```python
from build123d import *

# Parameters (mm, degrees)
SKETCH1_R           = 40
SKETCH1_W           = 12.2
SKETCH1_H           = 22.7
BOSS_EXTRUDE1_DEPTH = 16.35
SKETCH3_W           = 5
SKETCH3_H           = 34.105
CUT_EXTRUDE1_DEPTH  = 7
SKETCH4_R           = 1.75
CUT_EXTRUDE2_DEPTH  = 8
SKETCH2_R           = 40
SKETCH2_W           = 12.2
SKETCH2_H           = 32.25
BOSS_EXTRUDE2_DEPTH = 8.3
SKETCH5_R           = 1
CUT_EXTRUDE3_DEPTH  = 8
SKETCH6_R           = 40
BOSS_EXTRUDE3_DEPTH = 2.5
BOSS_EXTRUDE4_DEPTH = 31.05
CUT_EXTRUDE4_START  = -8
SKETCH8_R           = 1.75
CUT_EXTRUDE4_DEPTH  = 8
FILLET1_R           = 1


with BuildPart() as part:
    # Sketch1 → Boss-Extrude1 (new body)
    with BuildSketch(Plane(origin=(0, 0, 0), x_dir=(1, 0, 0), z_dir=(0, 1, 0))):
        with Locations(Location((0, 0, 0), (0, 0, 270))):
            Circle(SKETCH1_R)
        with Locations((0, 5.455)):
            Rectangle(SKETCH1_W, SKETCH1_H, mode=Mode.SUBTRACT)
    extrude(amount=BOSS_EXTRUDE1_DEPTH)

    # Sketch3 → Cut-Extrude1 (cut)
    with BuildSketch(Plane.XZ):
        with Locations((0, 22.9475)):
            Rectangle(SKETCH3_W, SKETCH3_H)
    extrude(amount=-CUT_EXTRUDE1_DEPTH, mode=Mode.SUBTRACT)

    # Sketch4 → Cut-Extrude2 (cut)
    with BuildSketch(Plane.XZ):
        with Locations(Location((-15.556349186, 15.556349186, 0), (0, 0, 270))):
            Circle(SKETCH4_R)
        with Locations(Location((15.556349186, 15.556349186, 0), (0, 0, 270))):
            Circle(SKETCH4_R)
        with Locations(Location((15.556349186, -15.556349186, 0), (0, 0, 270))):
            Circle(SKETCH4_R)
        with Locations(Location((-15.556349186, -15.556349186, 0), (0, 0, 270))):
            Circle(SKETCH4_R)
    extrude(amount=-CUT_EXTRUDE2_DEPTH, mode=Mode.SUBTRACT)

    # Sketch2 → Boss-Extrude2 (add)
    with BuildSketch(Plane(origin=(0, 16.35, 0), x_dir=(1, 0, 0), z_dir=(0, 1, 0))):
        with Locations(Location((0, 0, 0), (0, 0, 266.416678302))):
            Circle(SKETCH2_R)
        with Locations((0, 5.455)):
            Rectangle(SKETCH2_W, SKETCH2_H, mode=Mode.SUBTRACT)
    extrude(amount=BOSS_EXTRUDE2_DEPTH)

    # Sketch5 → Cut-Extrude3 (cut)
    with BuildSketch(Plane(origin=(0, 16.35, 0), x_dir=(1, 0, 0), z_dir=(0, 1, 0))):
        with Locations(Location((0, 19.58, 0), (0, 0, 270))):
            Circle(SKETCH5_R)
        with Locations(Location((0, -8.67, 0), (0, 0, 90))):
            Circle(SKETCH5_R)
    extrude(amount=-CUT_EXTRUDE3_DEPTH, mode=Mode.SUBTRACT)

    # Sketch6 → Boss-Extrude3 (add)
    with BuildSketch(Plane(origin=(0, 24.65, 0), x_dir=(1, 0, 0), z_dir=(0, 1, 0))):
        with Locations(Location((0, 0, 0), (0, 0, 266.416678302))):
            Circle(SKETCH6_R)
        with BuildLine():
            Line((6.1, 12.043255374), (6.1, 21.58))
            Line((6.1, 21.58), (-6.1, 21.58))
            Line((-6.1, 21.58), (-6.1, 12.043255374))
            ThreePointArc((-6.1, 12.043255374), (0, -13.5), (6.1, 12.043255374))
        make_face(mode=Mode.SUBTRACT)
    extrude(amount=BOSS_EXTRUDE3_DEPTH)

    # Sketch7 → Boss-Extrude4 (add)
    with BuildSketch(Plane(origin=(0, 27.15, 0), x_dir=(1, 0, 0), z_dir=(0, 1, 0))):
        with BuildLine():
            ThreePointArc((-4.790054945, -12.621623256), (-13.48100084, -0.715972321), (-6.1, 12.043255374))
            Line((-6.1, 12.043255374), (-6.1, 21.58))
            Line((-6.1, 21.58), (6.1, 21.58))
            Line((6.1, 21.58), (6.1, 12.043255374))
            ThreePointArc((6.1, 12.043255374), (13.480999281, -0.716001663), (4.79, -12.621644108))
            Line((4.79, -12.621644108), (4.79, -13))
            Line((4.79, -13), (10.89, -13))
            Line((10.89, -13), (10.89, -14.6))
            Line((10.89, -14.6), (7.39, -14.6))
            Line((7.39, -14.6), (7.39, -39.311422004))
            ThreePointArc((7.39, -39.311422004), (30.786360616, -25.538206672), (40, 0))
            ThreePointArc((40, 0), (-29.929918142, 26.536766947), (4.79, -39.712163124))
            Line((4.79, -39.712163124), (4.79, -14.6))
            Line((4.79, -14.6), (-6.11, -14.6))
            Line((-6.11, -14.6), (-6.11, -13))
            Line((-6.11, -13), (-4.790054945, -13))
            Line((-4.790054945, -13), (-4.790054945, -12.621623256))
        make_face()
    extrude(amount=BOSS_EXTRUDE4_DEPTH)

    # Sketch8 → Cut-Extrude4 (cut)
    with BuildSketch(Plane(origin=(0, 58.2, 0), x_dir=(1, 0, 0), z_dir=(0, 1, 0)).offset(CUT_EXTRUDE4_START)):
        with Locations(Location((-15.556349186, 15.556349186, 0), (0, 0, 90))):
            Circle(SKETCH8_R)
        with Locations(Location((15.556349186, 15.556349186, 0), (0, 0, 90))):
            Circle(SKETCH8_R)
        with Locations(Location((15.556349186, -15.556349186, 0), (0, 0, 90))):
            Circle(SKETCH8_R)
        with Locations(Location((-15.556349186, -15.556349186, 0), (0, 0, 90))):
            Circle(SKETCH8_R)
    extrude(amount=CUT_EXTRUDE4_DEPTH, mode=Mode.SUBTRACT)

    # Fillet1
    # the kernel refuses this fillet: 1 mm, written as the material it takes off along each edge
    with BuildSketch(Plane(origin=(-2.5, 7, 39.921798557), x_dir=(-0.9970979844940963, 0, -0.07612889936030137), z_dir=(0, -1, 0))) as fillet1_piece_1:
        with BuildLine():
            CenterArc((1.079253806, 0.999906678), FILLET1_R, 175.633911064, 95.148856173)
            Line((0.082155822, 1.076035578), (0, 0))
            ThreePointArc((0, 0), (0.546457623, -0.003732873), (1.092915247, 0))
        make_face()
    extrude(amount=9.732288117, mode=Mode.SUBTRACT)
    with BuildSketch(Plane(origin=(2.5, 7, 39.921798557), x_dir=(0.9970979844940963, 0, -0.07612889936030175), z_dir=(0, -1, 0))) as fillet1_piece_2:
        with BuildLine():
            CenterArc((1.079253806, -0.999906678), FILLET1_R, 89.217232763, 95.148856173)
            Line((0.082155822, -1.076035578), (0, 0))
            ThreePointArc((0, 0), (0.546457623, 0.003732873), (1.092915247, 0))
        make_face()
    extrude(amount=9.732288117, mode=Mode.SUBTRACT)
    with BuildSketch(Plane(origin=(0, 7, 0), x_dir=(0.12471521651868436, 0, 0.9921925794767352), z_dir=(0.9921925794767352, 0, -0.12471521651868436))) as fillet1_piece_3_section:
        with BuildLine():
            CenterArc((40 - FILLET1_R, -FILLET1_R), FILLET1_R, 0, 90)
            Line((40 - FILLET1_R, 0), (40, 0))
            Line((40, 0), (40, -FILLET1_R))
        make_face()
    fillet1_piece_3 = revolve(axis=Axis((0, 7, 0), (0, -1, 0)), revolution_arc=7.164310198, mode=Mode.PRIVATE)
    fillet1_piece_3 = split(fillet1_piece_3, bisect_by=Plane(origin=(2.5, 7.226394193, 39.747383267), z_dir=(-1, 0, 0)), keep=Keep.TOP, mode=Mode.PRIVATE)
    add(fillet1_piece_3, mode=Mode.SUBTRACT)
    with BuildSketch(Plane(origin=(0, 27.15, 0), x_dir=(0.057506279993827, 0, 0.9983451446074506), z_dir=(-0.9983451446074506, 0, 0.057506279993827))) as fillet1_piece_4_section:
        with BuildLine():
            CenterArc((40 - FILLET1_R, -FILLET1_R), FILLET1_R, 0, 90)
            Line((40 - FILLET1_R, 0), (40, 0))
            Line((40, 0), (40, -FILLET1_R))
        make_face()
    fillet1_piece_4 = revolve(axis=Axis((0, 27.15, 0), (0, 1, 0)), revolution_arc=10.930860095, mode=Mode.PRIVATE)
    fillet1_piece_4 = split(fillet1_piece_4, bisect_by=Plane(origin=(4.79, 26.923621973, 39.296870163), z_dir=(1, 0, 0)), keep=Keep.TOP, mode=Mode.PRIVATE)
    fillet1_piece_4 = split(fillet1_piece_4, bisect_by=Plane(origin=(7.39, 26.923621973, 39.296870163), z_dir=(-1, 0, 0)), keep=Keep.TOP, mode=Mode.PRIVATE)
    add(fillet1_piece_4, mode=Mode.SUBTRACT)
    with BuildSketch(Plane(origin=(0, 7, 0), x_dir=(0, 0, 1), z_dir=(1, 0, 0))) as fillet1_piece_5_section:
        with BuildLine():
            CenterArc((40 - FILLET1_R, -FILLET1_R), FILLET1_R, 0, 90)
            Line((40 - FILLET1_R, 0), (40, 0))
            Line((40, 0), (40, -FILLET1_R))
        make_face()
    fillet1_piece_5 = revolve(axis=Axis((0, 7, 0), (0, -1, 0)), revolution_arc=7.164310198, mode=Mode.PRIVATE)
    fillet1_piece_5 = split(fillet1_piece_5, bisect_by=Plane(origin=(-2.5, 7.226394086, 39.74738287), z_dir=(1, 0, 0)), keep=Keep.TOP, mode=Mode.PRIVATE)
    add(fillet1_piece_5, mode=Mode.SUBTRACT)
    with BuildSketch(Plane(origin=(0, 7, 0), x_dir=(0, 0, 1), z_dir=(1, 0, 0))) as fillet1_piece_6a_section:
        with BuildLine():
            CenterArc((40 - FILLET1_R, -FILLET1_R), FILLET1_R, 0, 90)
            Line((40 - FILLET1_R, 0), (40, 0))
            Line((40, 0), (40, -FILLET1_R))
        make_face()
    fillet1_piece_6a = revolve(axis=Axis((0, 7, 0), (0, -1, 0)), revolution_arc=7.164310198, mode=Mode.PRIVATE)
    fillet1_piece_6a = split(fillet1_piece_6a, bisect_by=Plane(origin=(-2.5, 7.227785013, 39.594106119), z_dir=(-1, 0, 0)), keep=Keep.TOP, mode=Mode.PRIVATE)
    with BuildSketch(Plane(origin=(-2.5, 9.732288117, 39.921798557), x_dir=(-0.9970979844940969, 0, -0.07612889936029517), z_dir=(0, -1, 0))) as fillet1_piece_6b_section:
        with BuildLine():
            CenterArc((1.079253806, 0.999906678), FILLET1_R, 175.633911064, 95.148856173)
            Line((0.082155822, 1.076035578), (0, 0))
            ThreePointArc((0, 0), (0.546457623, -0.003732873), (1.092915247, 0))
        make_face()
    fillet1_piece_6b = extrude(amount=12.464576234, mode=Mode.PRIVATE)
    fillet1_piece_6b = split(fillet1_piece_6b, bisect_by=Plane(origin=(-2.749431224, 7, 39.658633208), z_dir=(0, 1, 0)), keep=Keep.TOP, mode=Mode.PRIVATE)
    fillet1_piece_6 = fillet1_piece_6a & fillet1_piece_6b
    add(fillet1_piece_6, mode=Mode.SUBTRACT)
    with BuildSketch(Plane(origin=(2.5, 9.732288117, 39.921798557), x_dir=(0.9970979844940969, 0, -0.07612889936029532), z_dir=(0, -1, 0))) as fillet1_piece_7a_section:
        with BuildLine():
            CenterArc((1.079253806, -0.999906678), FILLET1_R, 89.217232763, 95.148856173)
            Line((0.082155822, -1.076035578), (0, 0))
            ThreePointArc((0, 0), (0.546457623, 0.003732873), (1.092915247, 0))
        make_face()
    fillet1_piece_7a = extrude(amount=12.464576234, mode=Mode.PRIVATE)
    fillet1_piece_7a = split(fillet1_piece_7a, bisect_by=Plane(origin=(2.749431224, 7, 39.658633208), z_dir=(0, 1, 0)), keep=Keep.TOP, mode=Mode.PRIVATE)
    with BuildSketch(Plane(origin=(0, 7, 0), x_dir=(0.12471521651868436, 0, 0.9921925794767352), z_dir=(0.9921925794767352, 0, -0.12471521651868436))) as fillet1_piece_7b_section:
        with BuildLine():
            CenterArc((40 - FILLET1_R, -FILLET1_R), FILLET1_R, 0, 90)
            Line((40 - FILLET1_R, 0), (40, 0))
            Line((40, 0), (40, -FILLET1_R))
        make_face()
    fillet1_piece_7b = revolve(axis=Axis((0, 7, 0), (0, -1, 0)), revolution_arc=7.164310198, mode=Mode.PRIVATE)
    fillet1_piece_7b = split(fillet1_piece_7b, bisect_by=Plane(origin=(2.5, 7.227784999, 39.594105903), z_dir=(1, 0, 0)), keep=Keep.TOP, mode=Mode.PRIVATE)
    fillet1_piece_7 = fillet1_piece_7a & fillet1_piece_7b
    add(fillet1_piece_7, mode=Mode.SUBTRACT)


solid = part.part
```
Verification items for the finished model (mm, model axes). A direction names the side the tool comes from. Coordinates: 2 decimals unless noted, no trailing zeros. Loops run counter-clockwise (first coordinate to the right, second up) from the corner with the lowest first, then second, coordinate; pieces in that order, holes last. Notation, with made-up numbers: (-15.75, -26.5) -> (3.25, -26.5) arc R26 cw to (3.25, 11.5) -> close; hole circle Ø6 at (-21, 54.5). An arc over 180 degrees is marked (long way). Answer in a Markdown table with one row per item. Add a question column.
1. Section check B-B, the plane y = 30. Enter the section's corners in (x, z), then the cut area to 3 significant figures.
2. Section check C-C, the plane x = -18.5. Enter the section's corners in (y, z).
3. Material ranges on probe 1 along Z at (x, y) = (0, 25.75); probe 2 along Y at (x, z) = (6.5, 7.5); probe 3 along X at (y, z) = (30, 31), recorded low to high. Write a range as [from, to].
4. Depth check by flat-ended pin: P1, Ø5, axis at y = 35.5, z = 9.5, coming from the -X side; P2, Ø2, axis at y = 44.5, z = 9, coming from the -X side; P3, Ø4, axis at y = 14, z = 7, coming from the +X side. Enter the tip coordinate at first touch or a pass-through.
5. Section check A-A, the plane z = -2. Enter the section's corners in (x, y), then the cut area to 3 significant figures.
6. Section check D-D, the plane y = 54.5. Enter the section's corners in (x, z).
7. Access from +Z, -Z, +X, -X, +Y, -Y to the whole of each face (thin tool, end or side, straight path). Record for faces 1 (the face through (-16, 8, -16)), 2 (the face through (16, 50.2, -16)), 3 (the face through (4.79, 42, 27)).
8. Draft check along Z on faces 4 (the face through (-16, 8, 16)), 5 (the face through (-16, 50.2, 16)), 6 (the face through (-2.5, 3, 22)). Enter one of: +Z half, -Z half, draft (parallel to the pull), parting line (faces both ways), or undercut.
Derived:
| question | item | result |
|---|---|---|
| 1 | outline | (-6.11, 13) -> (-6.11, 14.6) -> (4.79, 14.6) -> (4.79, 39.71) arc R40 ccw (long way) to (7.39, 39.31) -> (7.39, 14.6) -> (10.89, 14.6) -> (10.89, 13) -> (4.79, 13) -> (4.79, 12.62) arc R13.5 cw to (6.1, -12.04) -> (6.1, -21.58) -> (-6.1, -21.58) -> (-6.1, -12.04) arc R13.5 cw to (-4.79, 12.62) -> (-4.79, 13) -> close |
| 1 | area | 4,260 mm² |
| 2 | outline | (0, -35.46) -> (58.2, -35.46) -> (58.2, 35.46) -> (0, 35.46) -> close |
| 3 | probe 1 | z = [-40, -21.58], [13.5, 40] |
| 3 | probe 2 | y = [0, 24.65] |
| 3 | probe 3 | x = [-25.28, 4.79], [7.39, 25.28] |
| 4 | P1 | stops at x = -39.38 |
| 4 | P2 | stops at x = -39.19 |
| 4 | P3 | stops at x = 39.69 |
| 5 | outline | (-39.95, 0) -> (-6.1, 0) -> (-6.1, 24.65) -> (-13.35, 24.65) -> (-13.35, 58.2) -> (-39.95, 58.2) -> close; (6.1, 0) -> (39.95, 0) -> (39.95, 58.2) -> (13.35, 58.2) -> (13.35, 24.65) -> (6.1, 24.65) -> close |
| 5 | area | 3,450 mm² |
| 6 | outline | (-6.11, 13) -> (-6.11, 14.6) -> (4.79, 14.6) -> (4.79, 39.71) arc R40 ccw (long way) to (7.39, 39.31) -> (7.39, 14.6) -> (10.89, 14.6) -> (10.89, 13) -> (4.79, 13) -> (4.79, 12.62) arc R13.5 cw to (6.1, -12.04) -> (6.1, -21.58) -> (-6.1, -21.58) -> (-6.1, -12.04) arc R13.5 cw to (-4.79, 12.62) -> (-4.79, 13) -> close; hole circle Ø3.5 at (-15.56, -15.56); hole circle Ø3.5 at (-15.56, 15.56); hole circle Ø3.5 at (15.56, -15.56); hole circle Ø3.5 at (15.56, 15.56) |
| 7 | face 1 | -Y |
| 7 | face 2 | +Y |
| 7 | face 3 | +Z, +Y |
| 8 | face 4 | undercut |
| 8 | face 5 | undercut |
| 8 | face 6 | draft |
